from build123d import *

# Parameters (mm, degrees)
SKETCH_1_W        = 11.6
SKETCH_1_H        = 19.8
SKETCH_1_R        = 2.2
EXTRUDE_1_DEPTH   = 5
EXTRUDE_1_2_DEPTH = 5
SKETCH_3_W        = 64
SKETCH_3_H        = 30
SKETCH_3_R        = 1.65
EXTRUDE_2_DEPTH   = 4


with BuildPart() as part:
    # Sketch 1 → Extrude 1 (new body)
    with BuildSketch(Plane.XY):
        with Locations((26.2, -9.9)):
            Rectangle(SKETCH_1_W, SKETCH_1_H)
        with Locations((24, -4.9)):
            Circle(SKETCH_1_R, mode=Mode.SUBTRACT)
        with Locations(Location((24, -14.9, 0), (0, 0, 180))):
            Circle(SKETCH_1_R, mode=Mode.SUBTRACT)
    extrude(amount=EXTRUDE_1_DEPTH)



with BuildPart() as body_2:
    # Sketch 1 → Extrude 1 2 (new body)
    with BuildSketch(Plane.XY):
        with Locations((-26.2, -9.9)):
            Rectangle(SKETCH_1_W, SKETCH_1_H)
        with Locations((-24, -14.9)):
            Circle(SKETCH_1_R, mode=Mode.SUBTRACT)
        with Locations(Location((-24, -4.9, 0), (0, 0, 180))):
            Circle(SKETCH_1_R, mode=Mode.SUBTRACT)
    extrude(amount=EXTRUDE_1_2_DEPTH)


with BuildPart() as part_1:
    add(part.part)

    add(body_2.part)  # Extrude 2 merges body 2
    # Sketch 3 → Extrude 2 (add)
    with BuildSketch(Plane(origin=(0, 0, 0), x_dir=(1, 0, 0), z_dir=(0, 1, 0))):
        with Locations((0, -15)):
            Rectangle(SKETCH_3_W, SKETCH_3_H)
        with Locations(Location((-29, -15, 0), (0, 0, 270))):
            Circle(SKETCH_3_R, mode=Mode.SUBTRACT)
        with Locations(Location((-29, -25, 0), (0, 0, 270))):
            Circle(SKETCH_3_R, mode=Mode.SUBTRACT)
        with Locations(Location((29, -25, 0), (0, 0, 90))):
            Circle(SKETCH_3_R, mode=Mode.SUBTRACT)
        with Locations(Location((29, -15, 0), (0, 0, 90))):
            Circle(SKETCH_3_R, mode=Mode.SUBTRACT)
    extrude(amount=EXTRUDE_2_DEPTH)


solid = part_1.part
For this review, take the finished solid that the model builds, in its own axes (mm). A direction names the side the tool comes from. Round coordinates to 2 decimals unless told otherwise and drop trailing zeros. Order: outer loops, then holes, each group sorted by start corner. A loop starts at its lowest first (then second) coordinate and runs counter-clockwise, first axis right, second up. Notation, with made-up numbers: (-24, -30) -> (27, -30) arc R28 cw to (27, 4) -> close; hole circle Ø5 at (-2.5, 9). An arc over 180 degrees is marked (long way). Write item = value, one per line. Start each with the question number.
1) The part is to be moulded in two halves that separate along Z. For faces 6 (the face through (-27.885, 1.972, 23.784)), 7 (the face through (-20.4, -10, 2)), 8 (the face through (0, 2, 30)), 9 (the face through (-27.61, 1.97, 15.89)), say which applies: +Z half, -Z half, draft (parallel to the pull), parting line (faces both ways), or undercut.
2) To check wall thickness, follow line 1 (X direction, y = 1.6, z = 25); line 2 (Z direction, x = 29, y = 2.9); line 3 (Y direction, x = 9.5, z = 12.5). State the ranges of each line that lie inside material, in increasing order. Write a range as from..to.
3) Take a section at B-B on z = 15. State the section outline as (x, y) points.
4) Tool access review of faces 1 (the face through (20.4, -10, 2)), 2 (the face through (0, 3, 0)), 3 (the face through (-26, -19.8, 2)), 4 (the face through (0, 0, 15)), 5 (the face through (-26, -10, 5)): name each direction out of +Z, -Z, +X, -X, +Y, -Y from which nothing blocks a thin tool from reaching the whole face with its end or side.
5) Take a section at A-A on y = -12. State the section outline as (x, z) points.
6) Insertion check: pin 1 (3.5 mm diameter, centred on x = -25, y = -11, fed in from +Z); pin 2 (9 mm diameter, centred on x = 7.5, z = 19.5, fed in from -Y). Each pin has a flat end and moves straight along its axis. Give the tip position at first contact, or say it passes through.
7) Take a section at C-C on x = -24. State the section outline as (y, z) points, plus the area to 3 significant figures.
8) Take a section at D-D on y = 1.5. State the section outline as (x, z) points, plus the area to 3 significant figures.
Verdict:
q1.face_6 = undercut
q1.face_7 = draft
q1.face_8 = +Z half
q1.face_9 = undercut
q2.line_1 = -32..-30.65, -27.35..27.35, 30.65..32
q2.line_2 = 0..13.35, 16.65..23.35, 26.65..30
q2.line_3 = 0..4
q3.outline = (-32, 0) -> (-30.65, 0) -> (-30.65, 4) -> (-32, 4) -> close; (-27.35, 0) -> (27.35, 0) -> (27.35, 4) -> (-27.35, 4) -> close; (30.65, 0) -> (32, 0) -> (32, 4) -> (30.65, 4) -> close
q4.face_1 = +Z, -Z, -Y
q4.face_2 = -Z, +X, -X, +Y, -Y
q4.face_3 = +Z, -Z, +X, -X, -Y
q4.face_4 = +Z, -Y
q4.face_5 = +Z, +X, -X, -Y
q5.outline = (-32, 0) -> (-20.4, 0) -> (-20.4, 5) -> (-32, 5) -> close; (20.4, 0) -> (32, 0) -> (32, 5) -> (20.4, 5) -> close
q6.pin_1 = 5
q6.pin_2 = 0
q7.outline = (-19.8, 0) -> (-17.1, 0) -> (-17.1, 5) -> (-19.8, 5) -> close; (-12.7, 0) -> (-7.1, 0) -> (-7.1, 5) -> (-12.7, 5) -> close; (-2.7, 0) -> (4, 0) -> (4, 30) -> (0, 30) -> (0, 5) -> (-2.7, 5) -> close
q7.area = 175 mm2
q8.outline = (-32, 0) -> (32, 0) -> (32, 30) -> (-32, 30) -> close; hole circle Ø3.3 at (-29, 15); hole circle Ø3.3 at (-29, 25); hole circle Ø3.3 at (29, 15); hole circle Ø3.3 at (29, 25)
q8.area = 1,890 mm2
